Read the model definition and answer for the solid it produces. Units are mm, in the model's axes. Face numbers are marked on the shaded views. A direction names the side the tool comes from. Give positions to 0.01 mm unless a question says otherwise; leave off trailing zeros. Write each loop counter-clockwise with the first axis right and the second up, starting at its lowest first coordinate (ties: lowest second). Pieces come first, ordered by that corner, then holes.
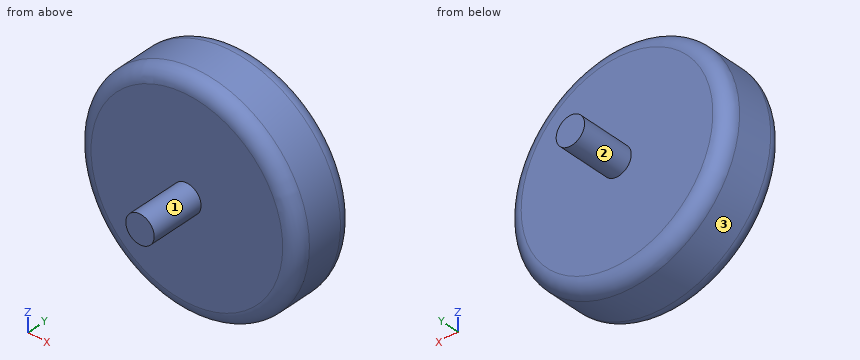
```python
from build123d import *

# Parameters (mm, degrees)
F0_R     = 3.175
F1_DEPTH = 38.1
F3_START = 11.8872
F2_R     = 24.60625
F3_DEPTH = 14.2748
F4_R     = 3.175
F5_R     = 3.175


with BuildPart() as f1:
    # F0 (on Front) → F1 (new body)
    with BuildSketch(Plane.XZ):
        Circle(F0_R)
    extrude(amount=F1_DEPTH)

    # F2 (on Front) → F3 (join)
    with BuildSketch(Plane.XZ.offset(F3_START)):
        Circle(F2_R)
    extrude(amount=F3_DEPTH)

    # F4
    f4_edges = [f1.edges().sort_by_distance(p)[0] for p in [
        (-24.60625, -26.162, 0),
    ]]
    fillet(f4_edges, radius=F4_R)

    # F5
    f5_edges = [f1.edges().sort_by_distance(p)[0] for p in [
        (-24.60625, -11.8872, 0),
    ]]
    fillet(f5_edges, radius=F5_R)


solid = f1.part
```
Item 1: Section A-A (x = 0) is taken. Write down the section's boundary in (y, z) (3 decimals).
Result set:
outline: (-38.1, -3.175) - (-26.162, -3.175) - (-26.162, -21.431) arc R3.175 ccw to (-22.987, -24.606) - (-15.062, -24.606) arc R3.175 ccw to (-11.887, -21.431) - (-11.887, -3.175) - (0, -3.175) - (0, 3.175) - (-11.887, 3.175) - (-11.887, 21.431) arc R3.175 ccw to (-15.062, 24.606) - (-22.987, 24.606) arc R3.175 ccw to (-26.162, 21.431) - (-26.162, 3.175) - (-38.1, 3.175) - close
Item 2: Each of these flat-tipped pins is pushed along its axis until it touches: pin 1 Ø8 at (y, z) = (-25, -2) entering from +X; pin 2 Ø1 at (x, z) = (1, -16.5) entering from +Y; pin 3 Ø8 at (y, z) = (-20, 18.5) entering from +X; pin 4 Ø12 at (x, z) = (5.5, 17) entering from -Y. Where does it stop, or does it pass through?
Result set:
pin 1: stops at x = 24.61
pin 2: stops at y = -11.89
pin 3: stops at x = 19.88
pin 4: stops at y = -26.16
Item 3: Find the intervals of material crossed by line 1 along Y through (x, z) = (14.5, 13); line 2 along X through (y, z) = (-12.5, 11); line 3 along X through (y, z) = (-24, -7.5), in increasing order.
Result set:
line 1: y = -26.16 to -11.89
line 2: x = -20.55 to 20.55
line 3: x = -23.26 to 23.26
Item 4: Section B-B (z = 0) is taken. Write down the section's boundary in (x, y) (3 decimals).
Result set:
outline: (-24.606, -22.987) arc R3.175 ccw to (-21.431, -26.162) - (-3.175, -26.162) - (-3.175, -38.1) - (3.175, -38.1) - (3.175, -26.162) - (21.431, -26.162) arc R3.175 ccw to (24.606, -22.987) - (24.606, -15.062) arc R3.175 ccw to (21.431, -11.887) - (3.175, -11.887) - (3.175, 0) - (-3.175, 0) - (-3.175, -11.887) - (-21.431, -11.887) arc R3.175 ccw to (-24.606, -15.062) - close
Item 5: Which of the six approach directions +Z, -Z, +X, -X, +Y, -Y give full straight-line access (tool end or side, diameter ignored) to the marked faces 1, 2 and 3?
Result set:
face 1: -Y
face 2: +Y
face 3: +Y, -Y
Item 6: Section D-D (y = -4) is taken. Write down the section's boundary in (x, z) (3 decimals).
Result set:
outline: circle Ø6.35 at (0, 0)
Item 7: Section C-C (y = -20) is taken. Write down the section's boundary in (x, z), and give its area (3 significant figures).
Result set:
outline: circle Ø49.21 at (0, 0)
area: 1,900 mm2
